CAD build for the part. Positions are in the model's coordinates, mm. Face numbers are marked on the shaded views. Give positions to 0.01 mm unless a question says otherwise; leave off trailing zeros. Order: outer loops, then holes, each group sorted by start corner. A loop starts at its lowest first (then second) coordinate and runs counter-clockwise, first axis right, second up. Notation, with made-up numbers: (62.25, 27.25) -> (97.25, 27.25) arc R9 cw to (97.25, 34.25) -> close; hole circle Ø6 at (23.5, -36). An arc over 180 degrees is marked (long way). Answer as CSV lines item,"result".
Autodesk Inventor part; units mm, degrees
ref_plane "YZ Plane" through (0, 0, 0) normal (1, 0, 0) x (0, 1, 0)
ref_plane "XZ Plane" through (0, 0, 0) normal (0, 1, 0) x (-1, 0, 0)
ref_plane "XY Plane" through (0, 0, 0) normal (0, 0, 1) x (1, 0, 0)
sketch "Sketch1" plane through (0, 0, 0) normal (0, 1, 0) x (-1, 0, 0)
  line L0 (0, 0) -> (28, 0)
  line L1 (28, 0) -> (28, -60)
  line L2 (28, -60) -> (0, -60)
  line L3 (0, -60) -> (0, 0)
  dimension "d0" = 60
  dimension "d1" = 28
extrude "Extrusion1" add sketch "Sketch1" along normal blind 27
sketch "Sketch2" plane through (0, 27, 0) normal (0, 1, 0) x (1, 0, 0)
  line L0 (0, 0) -> (0, 60)
  line L1 (0, 0) -> (-28, 0)
  line L2 (-28, 0) -> (-28, 30)
  line L3 (-28, 30) -> (0, 30)
  line L4 (0, 30) -> (0, 0)
  line L5 (-28, 60) -> (-28, 0)
  dimension "d4" = 30
extrude "Extrusion2" add sketch "Sketch2" along normal blind 5
sketch "Sketch3" plane through (0, 32, 0) normal (0, 1, 0) x (1, 0, 0)
  circle A0 centre (-14, 15) radius 7.5
  line L0 (0, 30) -> (-28, 30) construction
  line L1 (-28, 0) -> (0, 0) construction
  line L2 (0, 0) -> (0, 30) construction
  line L3 (0, 30) -> (-28, 30) construction
  line L4 (-28, 30) -> (-28, 0) construction
  line L5 (-28, 0) -> (0, 0) construction
  line L6 (-28, 30) -> (-28, 0) construction
  line L7 (-14, 0) -> (-14, 30) construction
  line L8 (-28, 15) -> (0, 15) construction
  line L9 (0, 60) -> (0, 0) construction
  point P0 (-14, 15)
  point P1 (-14, 15)
  dimension "d7" = 15
extrude "Extrusion3" cut sketch "Sketch3" against normal blind 5
sketch "Sketch4" plane through (0, 0, 0) normal (0, -1, 0) x (1, 0, 0)
  circle A0 centre (-2, -30) radius 1
  line L0 (0, -60) -> (0, 0)
  line L1 (0, -30) -> (0, -60)
  line L2 (0, -30) -> (-52.148, -30)
  line L3 (0, -30) -> (-28, -30)
  dimension "d10" = 2
  dimension "d11" = 2
extrude "Extrusion4" add sketch "Sketch4" along normal blind 5
sketch "Sketch5" plane through (-2, -5, -30) normal (0, -1, 0) x (1, 0, 0)
  circle A0 centre (0, 0) radius 1
  point P0 (2, 30)
properties part number "camera"
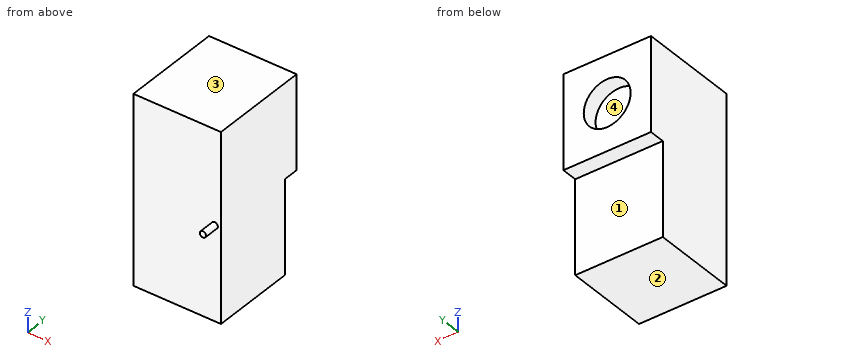
1) Band-saw the part on C-C, the plane x = -2. Write the cut outline in (y, z).
Data:
outline,"(-5, -31) -> (0, -31) -> (0, -60) -> (27, -60) -> (27, -30) -> (32, -30) -> (32, 0) -> (0, 0) -> (0, -29) -> (-5, -29) -> close"
2) Band-saw the part on B-B, the plane z = -15. Write the cut outline in (x, y), then the cut area to 3 significant figures.
Data:
outline,"(-28, 0) -> (0, 0) -> (0, 32) -> (-6.5, 32) -> (-6.5, 27) -> (-21.5, 27) -> (-21.5, 32) -> (-28, 32) -> close"
area,"821 mm2"
3) Pin check, flat tip, straight feed: P1, Ø2, axis at x = -5, z = -51.5, coming from the +Y side. Stop position of the tip, or through.
Data:
P1,"stops at y = 27"
4) Band-saw the part on A-A, the plane x = -14. Write the cut outline in (y, z).
Data:
outline,"(0, -60) -> (27, -60) -> (27, -30) -> (32, -30) -> (32, -22.5) -> (27, -22.5) -> (27, -7.5) -> (32, -7.5) -> (32, 0) -> (0, 0) -> close"
5) Pull direction Z, two halves, no side cores. Call the marked faces 1, 2, 3 and 4: pulls with the +Z half, pulls with the -Z half, needs draft (parallel to the pull), parting line crosses it, or undercut.
Data:
face 1,"needs draft"
face 2,"pulls with the -Z half"
face 3,"pulls with the +Z half"
face 4,"undercut"
6) Wall check: line 1 along Z through (x, y) = (-14, 29.1); line 2 along X through (y, z) = (28.1, -15); line 3 along Y through (x, z) = (-4.5, -25). Give the ranges that are in metal, low to high. Write a range as [from, to].
Data:
line 1,"z = [-30, -22.5], [-7.5, 0]"
line 2,"x = [-28, -21.5], [-6.5, 0]"
line 3,"y = [0, 32]"
7) Band-saw the part on D-D, the plane z = -41. Write the cut outline in (x, y), then the cut area to 3 significant figures.
Data:
outline,"(-28, 0) -> (0, 0) -> (0, 27) -> (-28, 27) -> close"
area,"756 mm2"
